Part model, mm, in its own coordinate system. A direction names the side the tool comes from. Give positions to 0.01 mm unless a question says otherwise; leave off trailing zeros. Order: outer loops, then holes, each group sorted by start corner. A loop starts at its lowest first (then second) coordinate and runs counter-clockwise, first axis right, second up. Notation, with made-up numbers: M 62.25,-21.75 L 115.25,-21.75 A14 ccw 115.25,5.25 Z; hole C 2,26 d7. An arc over 180 degrees is marked long. Answer as a JSON object with one key per item and string values.
from build123d import *

# Parameters (mm, degrees)
SKETCH_R     = 2.55
PAD_DEPTH    = 4.5
PAD001_DEPTH = 24
PAD002_DEPTH = 2
SKETCH004_R  = 4.5
POCKET_DEPTH = 3
FILLET_R     = 2.9


with BuildPart() as part:
    # Sketch → Pad (new body)
    with BuildSketch(Plane.XZ):
        with BuildLine():
            Line((-36, 5), (-36, 0))
            ThreePointArc((-36, 0), (0, -36), (36, 0))
            Line((36, 5), (36, 0))
            ThreePointArc((36, 5), (30, 11), (24, 5))
            Line((-24, 5), (24, 5))
            ThreePointArc((-24, 5), (-30, 11), (-36, 5))
        make_face()
        with Locations((-30, 5)):
            Circle(SKETCH_R, mode=Mode.SUBTRACT)
        with Locations((30, 5)):
            Circle(SKETCH_R, mode=Mode.SUBTRACT)
    extrude(amount=PAD_DEPTH)

    # Sketch002 (on Face10 of Pad) → Pad001 (join)
    with BuildSketch(Plane.XZ.offset(4.5)):
        with BuildLine():
            ThreePointArc((-33, 0), (0, -33), (33, 0))
            Line((29, 0), (33, 0))
            ThreePointArc((-29, 0), (0, -29), (29, 0))
            Line((-33, 0), (-29, 0))
        make_face()
    extrude(amount=PAD001_DEPTH)

    # Sketch003 (on Face15 of Pad001) → Pad002 (join)
    with BuildSketch(Plane.XZ.offset(28.5)):
        with BuildLine():
            ThreePointArc((-33, 0), (0, -33), (33, 0))
            ThreePointArc((33, 0), (27, 3), (21, 0))
            ThreePointArc((-21, 0), (0, -21), (21, 0))
            ThreePointArc((-21, 0), (-27, 3), (-33, 0))
        make_face()
    extrude(amount=PAD002_DEPTH)

    # Sketch004 (on Face10 of Pad) → Pocket (cut)
    with BuildSketch(Plane.XZ.offset(4.5)):
        with Locations((-30, 5)):
            Circle(SKETCH004_R)
        with Locations((30, 5)):
            Circle(SKETCH004_R)
    extrude(amount=-POCKET_DEPTH, mode=Mode.SUBTRACT)

    # Fillet
    fillet_edges = [part.edges().sort_by_distance(p)[0] for p in [
        (0, -4.5, -33),
    ]]
    fillet(fillet_edges, radius=FILLET_R)


solid = part.part
1. Two-plate mould, pull along Z, no slides. Class faces 5 (the cylindrical face through (-32.548, -0.74, 5.112)), 6 (the flat face through (-36, -2, 3)), 7 (the cylindrical face through (-0.79, -2.22, -35.99)): +Z half, -Z half, draft (parallel to the pull), parting line (faces both ways), or undercut.
Worked answers:
{"face 5": "undercut", "face 6": "draft", "face 7": "-Z half"}
2. Which spindle directions (+Z, -Z, +X, -X, +Y, -Y) get a long thin tool onto all of the face, cutting with end or side? Do faces 1 (the cylindrical face through (-0.638, -16.332, -28.993)), 2 (the flat face through (31, -16, 0)), 3 (the flat face through (-28, -1.5, 3)), 4 (the cylindrical face through (27, -29, 3)). Say none if no direction does.
Worked answers:
{"face 1": "+Z", "face 2": "+Z, +X, -X", "face 3": "none", "face 4": "+Z, -Y"}
3. Pin check, flat tips, straight feed: P1, Ø8, axis at x = 30, z = 5, coming from the +Y side; P2, Ø1, axis at x = -26, y = -6.5, coming from the +Z side; P3, Ø5, axis at x = 12, y = -2.5, coming from the +Z side; P4, Ø8, axis at y = -13, z = -30, coming from the -X side. Stop position of each tip, or through.
Worked answers:
{"P1": "stops at y = 0", "P2": "stops at z = -11.78", "P3": "stops at z = 5", "P4": "stops at x = -20.32"}
4. Cut at B-B on y = -15. Give the cut face in (x, z), plus the area to 3 significant figures.
Worked answers:
{"outline": "M -33,0 A33 ccw 33,0 L 29,0 A29 cw -29,0 Z", "area": "390 mm^2"}
5. Cut at A-A on x = 0. Give the cut face in (y, z).
Worked answers:
{"outline": "M -30.5,-33 L -7.4,-33 A2.9 cw -4.5,-35.9 L -4.5,-36 L 0,-36 L 0,5 L -4.5,5 L -4.5,-29 L -28.5,-29 L -28.5,-21 L -30.5,-21 Z"}
6. Probe line 1 along Y through (x, z) = (23.5, -2); line 2 along Y through (x, z) = (-29, 2.5); line 3 along Z through (x, y) = (30, -0.9). List the from-to ranges inside material, lowest first.
Worked answers:
{"line 1": "y = -30.5 to -28.5, -4.5 to 0", "line 2": "y = -30.5 to -28.5, -1.5 to 0", "line 3": "z = -19.9 to 2.45, 7.55 to 11"}
